Build history of the part. All positions in model axes, mm. Round coordinates to 2 decimals unless told otherwise and drop trailing zeros. Write each loop counter-clockwise with the first axis right and the second up, starting at its lowest first coordinate (ties: lowest second). Pieces come first, ordered by that corner, then holes. Notation, with made-up numbers: M 12.5,36 L 47.5,36 A14 ccw 47.5,48 Z; hole C -29,47 d11. An arc over 180 degrees is marked long. Write item = value, one per line.
from build123d import *

# Parameters (mm, degrees)
SKETCH1_W           = 300
SKETCH1_H           = 85
BOSS_EXTRUDE1_DEPTH = 3
SKETCH2_W           = 40
SKETCH2_H           = 3
CUT_EXTRUDE1_DEPTH  = 3
SKETCH3_W           = 40
SKETCH3_H           = 3
CUT_EXTRUDE2_DEPTH  = 3
SKETCH4_W           = 40
SKETCH4_H           = 3
CUT_EXTRUDE3_DEPTH  = 3
SKETCH5_W           = 40
SKETCH5_H           = 3
CUT_EXTRUDE4_DEPTH  = 3
SKETCH6_W           = 64
SKETCH6_H           = 23
CUT_EXTRUDE6_DEPTH  = 3
SKETCH7_W           = 64
SKETCH7_H           = 23
CUT_EXTRUDE7_DEPTH  = 3


with BuildPart() as part:
    # Sketch1 → Boss-Extrude1 (new body)
    with BuildSketch(Plane(origin=(0, 0, 0), x_dir=(1, 0, 0), z_dir=(0, 1, 0))):
        with Locations((-150, 42.5)):
            Rectangle(SKETCH1_W, SKETCH1_H)
    extrude(amount=BOSS_EXTRUDE1_DEPTH)

    # Sketch2 → Cut-Extrude1 (cut)
    with BuildSketch(Plane(origin=(0, 3, 0), x_dir=(1, 0, 0), z_dir=(0, 1, 0))):
        with Locations((-270, 4.5)):
            Rectangle(SKETCH2_W, SKETCH2_H)
    extrude(amount=-CUT_EXTRUDE1_DEPTH, mode=Mode.SUBTRACT)

    # Sketch3 → Cut-Extrude2 (cut)
    with BuildSketch(Plane(origin=(0, 3, 0), x_dir=(1, 0, 0), z_dir=(0, 1, 0))):
        with Locations((-30, 4.5)):
            Rectangle(SKETCH3_W, SKETCH3_H)
    extrude(amount=-CUT_EXTRUDE2_DEPTH, mode=Mode.SUBTRACT)

    # Sketch4 → Cut-Extrude3 (cut)
    with BuildSketch(Plane(origin=(0, 3, 0), x_dir=(1, 0, 0), z_dir=(0, 1, 0))):
        with Locations((-30, 80.5)):
            Rectangle(SKETCH4_W, SKETCH4_H)
    extrude(amount=-CUT_EXTRUDE3_DEPTH, mode=Mode.SUBTRACT)

    # Sketch5 → Cut-Extrude4 (cut)
    with BuildSketch(Plane(origin=(0, 3, 0), x_dir=(1, 0, 0), z_dir=(0, 1, 0))):
        with Locations((-270, 80.5)):
            Rectangle(SKETCH5_W, SKETCH5_H)
    extrude(amount=-CUT_EXTRUDE4_DEPTH, mode=Mode.SUBTRACT)

    # Sketch6 → Cut-Extrude6 (cut)
    with BuildSketch(Plane(origin=(0, 3, 0), x_dir=(1, 0, 0), z_dir=(0, 1, 0))):
        with Locations((-268, 17.5)):
            Rectangle(SKETCH6_W, SKETCH6_H)
    extrude(amount=-CUT_EXTRUDE6_DEPTH, mode=Mode.SUBTRACT)

    # Sketch7 → Cut-Extrude7 (cut)
    with BuildSketch(Plane(origin=(0, 3, 0), x_dir=(1, 0, 0), z_dir=(0, 1, 0))):
        with Locations((-32, 17.5)):
            Rectangle(SKETCH7_W, SKETCH7_H)
    extrude(amount=-CUT_EXTRUDE7_DEPTH, mode=Mode.SUBTRACT)


solid = part.part
1. Band-saw the part on C-C (z = -11.5). List the corners of the cut face in (x, y), plus the area to 3 significant figures.
Responses:
outline = M -236,0 L -64,0 L -64,3 L -236,3 Z
area = 516 mm²
2. Band-saw the part on B-B (y = 1.35). List the corners of the cut face in (x, z).
Responses:
outline = M -300,-85 L 0,-85 L 0,-29 L -64,-29 L -64,-6 L -50,-6 L -50,-3 L -10,-3 L -10,-6 L 0,-6 L 0,0 L -300,0 L -300,-6 L -290,-6 L -290,-3 L -250,-3 L -250,-6 L -236,-6 L -236,-29 L -300,-29 Z; hole M -290,-82 L -250,-82 L -250,-79 L -290,-79 Z; hole M -50,-82 L -10,-82 L -10,-79 L -50,-79 Z
3. Probe probe 1 along Z at (x, y) = (-12.5, 1); probe 2 along X at (y, z) = (1.75, -5.5); probe 3 along Z at (x, y) = (-239.5, 1.8). List the from-to ranges inside material, lowest first.
Responses:
probe_1 = -85 to -82, -79 to -29, -3 to 0
probe_2 = -300 to -290, -250 to -50, -10 to 0
probe_3 = -85 to -29, -6 to 0
4. Band-saw the part on A-A (x = -271). List the corners of the cut face in (y, z).
Responses:
outline = M 0,-85 L 3,-85 L 3,-82 L 0,-82 Z; M 0,-79 L 3,-79 L 3,-29 L 0,-29 Z; M 0,-3 L 3,-3 L 3,0 L 0,0 Z
5. Flat gauge pin, fed straight in: pin 1 (0.9 mm diameter, centred on y = 1.5, z = -22, fed in from -X). Where does the tip first touch, or does it go through?
Responses:
pin_1 = -236
